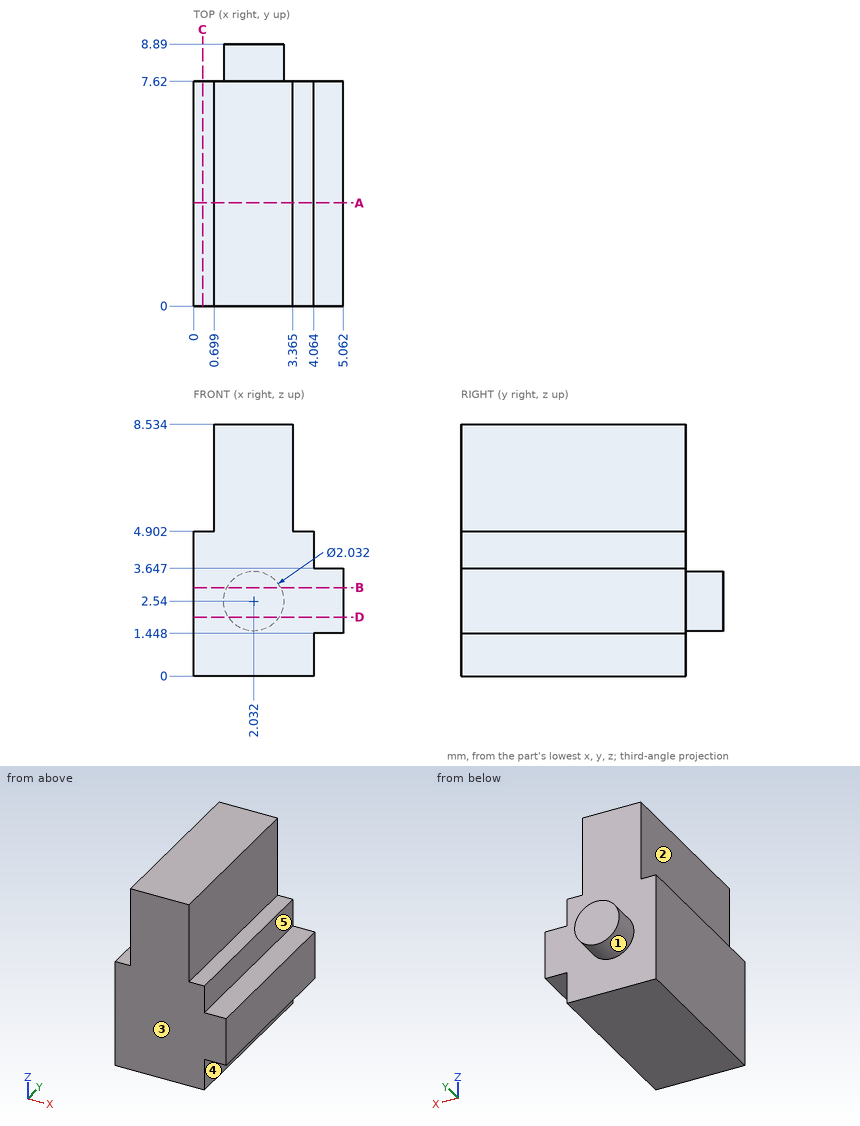
Answer from the drawing. Dimensions are ordinates in mm from the lowest x, y and z of the part. A direction names the side the tool comes from. Coordinates: 2 decimals unless noted, no trailing zeros. Write each loop counter-clockwise with the first axis right and the second up, starting at its lowest first coordinate (ties: lowest second). Pieces come first, ordered by that corner, then holes. Notation, with made-up numbers: (-30.5, -5.5) - (-19.5, -5.5) arc R12 ccw to (-19.5, 4.5) - close; hole circle Ø8 at (13, 0.25). An arc over 180 degrees is marked (long way). Return JSON: item names as keys, results as strings.
1. The part is cut by section D-D on z = 2. Determine the outline of the cut face in (x, y).
Final values:
{"outline": "(0, 0) - (5.06, 0) - (5.06, 7.62) - (2.89, 7.62) - (2.89, 8.89) - (1.17, 8.89) - (1.17, 7.62) - (0, 7.62) - close"}
2. The part is cut by section C-C on x = 0.3. Determine the outline of the cut face in (y, z).
Final values:
{"outline": "(0, 0) - (7.62, 0) - (7.62, 4.9) - (0, 4.9) - close"}
3. Consider line 1 along X through (y, z) = (2.75, 6.5) (1 decimal); line 2 along Z through (x, y) = (0.6, 1); line 3 along X through (y, z) = (2.25, 4.75) (1 decimal). Determine where each line is inside the solid, lowest interval first.
Final values:
{"line 1": "0.7 to 3.4", "line 2": "0 to 4.9", "line 3": "0 to 4.1"}
4. Which of the six approach directions +Z, -Z, +X, -X, +Y, -Y give full straight-line access (tool end or side, diameter ignored) to the marked faces 1, 2, 3, 4 and 5?
Final values:
{"face 1": "+Y", "face 2": "+Z, -X, +Y, -Y", "face 3": "+Z, -Z, +X, -X, -Y", "face 4": "-Z, +X, +Y, -Y", "face 5": "+Z, +X, +Y, -Y"}
5. The part is cut by section A-A on y = 3.5. Determine the outline of the cut face in (x, z) (1 decimal).
Final values:
{"outline": "(0, 0) - (4.1, 0) - (4.1, 1.4) - (5.1, 1.4) - (5.1, 3.6) - (4.1, 3.6) - (4.1, 4.9) - (3.4, 4.9) - (3.4, 8.5) - (0.7, 8.5) - (0.7, 4.9) - (0, 4.9) - close"}
6. The part is cut by section B-B on z = 3. Determine the outline of the cut face in (x, y).
Final values:
{"outline": "(0, 0) - (5.06, 0) - (5.06, 7.62) - (2.94, 7.62) - (2.94, 8.89) - (1.13, 8.89) - (1.13, 7.62) - (0, 7.62) - close"}
7. Each of these flat-tipped pins is pushed along its axis until it touches: pin 1 Ø1.1 at (y, z) = (4.5, 7) entering from -X; pin 2 Ø0.8 at (x, y) = (5, 5) entering from -Z; pin 3 Ø1.4 at (y, z) = (4.5, 4.5) entering from +X. Where does it stop, or does it pass through?
Final values:
{"pin 1": "x = 0.7", "pin 2": "z = 1.45", "pin 3": "x = 4.06"}
